Part model, mm, in its own coordinate system. Coordinates: 2 decimals unless noted, no trailing zeros. Write each loop counter-clockwise with the first axis right and the second up, starting at its lowest first coordinate (ties: lowest second). Pieces come first, ordered by that corner, then holes. Notation, with made-up numbers: M 52.25,64 L 56.25,64 A21 cw 56.25,85 Z; hole C 0,66 d3. An arc over 180 degrees is marked long. Use a Markdown table: item, result. Add a question column.
Q1. Slice it at A-A on y = -25. Write the cut outline in (x, z) (3 decimals), then the cut area to 3 significant figures.
Q2. Pin check, flat tips, straight feed: pin 1 Ø1.6 at (x, z) = (0.5, 2) entering from +Y; pin 2 Ø1.6 at (y, z) = (-39, 1) entering from +X; pin 3 Ø1 at (y, z) = (65, 1.5) entering from -X; pin 4 Ø10 at (x, y) = (7, 2.5) entering from -Z. Stop position of each tip, or through.
Q3. Wall check: L1, parallel to Y at x = 30, z = 0.8; L2, parallel to Y at x = -22, z = 1.8; L3, parallel to Y at x = 17, z = 2. Give the ranges that are in metal, low to high. Write a range as from..to.
Q4. Slice it at C-C on y = 33.5. Write the cut outline in (x, z) (3 decimals).
Q5. Slice it at B-B on x = 33. Write the cut outline in (y, z) (3 decimals), then the cut area to 3 significant figures.
Q6. Slice it at D-D on z = 2.3. Count the separate pieces of the cut face and the enclosed holes in it, then the cut area to 3 significant figures.
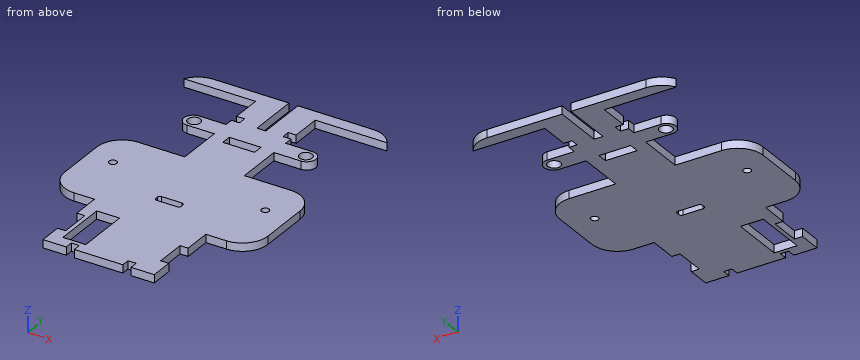
from build123d import *

# Parameters (mm, degrees)
SKETCH1_R           = 2.5
BOSS_EXTRUDE1_DEPTH = 3.175
FILLET1_R           = 10
SKETCH2_W           = 9
SKETCH2_H           = 21
CUT_EXTRUDE1_DEPTH  = 90.108082017
SKETCH3_W           = 12.5
SKETCH3_H           = 4
SKETCH3_W_2         = 3.5
SKETCH3_H_2         = 20
CUT_EXTRUDE2_DEPTH  = 90.108082017
FILLET2_R           = 10
SKETCH4_W           = 3.175
SKETCH4_H           = 3.175
BOSS_EXTRUDE2_DEPTH = 29
SKETCH5_W           = 3.175
SKETCH5_H           = 3.175
BOSS_EXTRUDE3_DEPTH = 29
SKETCH7_R           = 1.5
CUT_EXTRUDE3_DEPTH  = 10


with BuildPart() as part:
    # Sketch1 → Boss-Extrude1 (new body)
    with BuildSketch(Plane.XY):
        with BuildLine():
            Line((-9.56, -38.262636689), (-9.56, -41.437636689))
            Line((-9.56, -41.437636689), (9.56, -41.437636689))
            Line((9.56, -41.437636689), (9.56, -38.262636689))
            Line((9.56, -38.262636689), (12.735, -38.262636689))
            Line((12.735, -38.262636689), (12.735, -41.437636689))
            Line((12.735, -41.437636689), (15.91, -41.437636689))
            Line((15.91, -41.437636689), (21.91, -41.437636689))
            Line((21.91, -41.437636689), (21.91, -32.437636689))
            Line((21.91, -32.437636689), (18.735, -32.437636689))
            Line((18.735, -32.437636689), (18.735, -20.437636689))
            Line((18.735, -20.437636689), (21.91, -20.437636689))
            Line((21.91, -20.437636689), (21.91, -9.437636689))
            Line((21.91, -9.437636689), (40, -9.437636689))
            Line((40, -9.437636689), (40, 30.562363311))
            Line((40, 30.562363311), (10, 30.562363311))
            Line((10, 30.562363311), (10, 45.562363311))
            Line((10, 45.562363311), (10, 48.89577614))
            Line((10, 48.89577614), (22.410269523, 48.89577614))
            ThreePointArc((22.410269523, 48.89577614), (26.000000001, 52.562363311), (22.410269523, 56.228950483))
            Line((22.410269523, 56.228950483), (11.727794547, 56.228950483))
            Line((11.727794547, 56.228950483), (11.727794547, 59.562363311))
            Line((11.727794547, 59.562363311), (10, 59.562363311))
            Line((10, 59.562363311), (8.552794547, 59.562363311))
            Line((8.552794547, 59.562363311), (8.552794547, 62.737363311))
            Line((8.552794547, 62.737363311), (11.727794547, 62.737363311))
            Line((11.727794547, 62.737363311), (11.727794547, 74.562363311))
            Line((11.727794547, 74.562363311), (40, 74.562363311))
            Line((40, 74.562363311), (40, 79.562363311))
            Line((40, 79.562363311), (0, 79.562363311))
            Line((0, 79.562363311), (-40, 79.562363311))
            Line((-40, 79.562363311), (-40, 74.562363311))
            Line((-40, 74.562363311), (-11.727794547, 74.562363311))
            Line((-11.727794547, 74.562363311), (-11.727794547, 62.737363311))
            Line((-11.727794547, 62.737363311), (-8.552794547, 62.737363311))
            Line((-8.552794547, 62.737363311), (-8.552794547, 59.562363311))
            Line((-8.552794547, 59.562363311), (-10, 59.562363311))
            Line((-10, 59.562363311), (-11.727794547, 59.562363311))
            Line((-11.727794547, 59.562363311), (-11.727794547, 56.228950483))
            Line((-11.727794547, 56.228950483), (-22.410269523, 56.228950483))
            ThreePointArc((-22.410269523, 56.228950483), (-26.000000001, 52.562363311), (-22.410269523, 48.89577614))
            Line((-22.410269523, 48.89577614), (-10, 48.89577614))
            Line((-10, 48.89577614), (-10, 45.562363311))
            Line((-10, 45.562363311), (-10, 30.562363311))
            Line((-10, 30.562363311), (-40, 30.562363311))
            Line((-40, 30.562363311), (-40, -9.437636689))
            Line((-40, -9.437636689), (-21.91, -9.437636689))
            Line((-21.91, -9.437636689), (-21.91, -20.437636689))
            Line((-21.91, -20.437636689), (-18.735, -20.437636689))
            Line((-18.735, -20.437636689), (-18.735, -32.437636689))
            Line((-18.735, -32.437636689), (-21.91, -32.437636689))
            Line((-21.91, -32.437636689), (-21.91, -41.437636689))
            Line((-21.91, -41.437636689), (-15.91, -41.437636689))
            Line((-15.91, -41.437636689), (-12.735, -41.437636689))
            Line((-12.735, -41.437636689), (-12.735, -38.262636689))
            Line((-12.735, -38.262636689), (-9.56, -38.262636689))
        make_face()
        with BuildLine():
            Line((4, 1), (-4, 1))
            ThreePointArc((-4, 1), (-4.707106781, 1.292893219), (-5, 2))
            Line((-5, 2), (-5, 3))
            ThreePointArc((-5, 3), (-4.707106781, 3.707106781), (-4, 4))
            Line((-4, 4), (4, 4))
            ThreePointArc((4, 4), (4.707106781, 3.707106781), (5, 3))
            Line((5, 3), (5, 2))
            ThreePointArc((5, 2), (4.707106781, 1.292893219), (4, 1))
        make_face(mode=Mode.SUBTRACT)
        with Locations((-22, 52.562363311)):
            Circle(SKETCH1_R, mode=Mode.SUBTRACT)
        with Locations((22, 52.562363311)):
            Circle(SKETCH1_R, mode=Mode.SUBTRACT)
    extrude(amount=BOSS_EXTRUDE1_DEPTH)

    # Fillet1
    # the kernel refuses this fillet: 10 mm, written as the material it takes off along each edge
    with BuildSketch(Plane(origin=(-40, 79.562363311, -21.650635095), x_dir=(0, -1, 0), z_dir=(0, 0, 1))) as fillet1_piece_1:
        with BuildLine():
            CenterArc((10, 8.660254038), FILLET1_R, 180, 60)
            Line((0, 8.660254038), (-0.2, 8.660254038))
            Line((-0.2, 8.660254038), (-0.2, 0))
            Line((-0.2, 0), (0, -0.2))
            ThreePointArc((0, -0.2), (2.5, -0.2), (4.9, -0.173205081))
            Line((4.9, -0.173205081), (5, 0))
        make_face()
    extrude(amount=46.476270189, mode=Mode.SUBTRACT)
    with BuildSketch(Plane(origin=(40, 79.562363311, -21.650635095), x_dir=(-1, 0, 0), z_dir=(0, 0, 1))) as fillet1_piece_2:
        with BuildLine():
            CenterArc((8.660254038, 10), FILLET1_R, 210, 60)
            Line((0, 5), (-0.173205081, 4.9))
            ThreePointArc((-0.173205081, 4.9), (-0.2, 2.5), (-0.2, 0))
            Line((-0.2, 0), (0, -0.2))
            Line((0, -0.2), (8.660254038, -0.2))
            Line((8.660254038, -0.2), (8.660254038, 0))
        make_face()
    extrude(amount=46.476270189, mode=Mode.SUBTRACT)

    # Sketch2 → Cut-Extrude1 (cut, through all)
    with BuildSketch(Plane.XY.offset(3.175)):
        with Locations((-12.61, -26.137636689)):
            Rectangle(SKETCH2_W, SKETCH2_H)
    extrude(amount=-CUT_EXTRUDE1_DEPTH, mode=Mode.SUBTRACT)

    # Sketch3 → Cut-Extrude2 (cut, through all)
    with BuildSketch(Plane.XY.offset(3.175)):
        with Locations((0, 47.562363311)):
            Rectangle(SKETCH3_W, SKETCH3_H)
        with Locations((0, 69.663077344)):
            Rectangle(SKETCH3_W_2, SKETCH3_H_2)
    extrude(amount=-CUT_EXTRUDE2_DEPTH, mode=Mode.SUBTRACT)

    # Fillet2
    fillet2_edges = [part.edges().sort_by_distance(p)[0] for p in [
        (40, 30.562363311, 1.5875),
        (40, -9.437636689, 1.5875),
        (-40, -9.437636689, 1.5875),
        (-40, 30.562363311, 1.5875),
    ]]
    fillet(fillet2_edges, radius=FILLET2_R)

    # Sketch4 → Boss-Extrude2 (add)
    with BuildSketch(Plane(origin=(0, 59.562363311, 0), x_dir=(1, 0, 0), z_dir=(0, 1, 0))):
        with Locations((10.140294547, -1.5875)):
            Rectangle(SKETCH4_W, SKETCH4_H)
    extrude(amount=-BOSS_EXTRUDE2_DEPTH)

    # Sketch5 → Boss-Extrude3 (add)
    with BuildSketch(Plane(origin=(0, 59.562363311, 0), x_dir=(1, 0, 0), z_dir=(0, 1, 0))):
        with Locations((-10.140294547, -1.5875)):
            Rectangle(SKETCH5_W, SKETCH5_H)
    extrude(amount=-BOSS_EXTRUDE3_DEPTH)

    # Sketch7 → Cut-Extrude3 (cut)
    with BuildSketch(Plane.XY.offset(3.175)):
        with Locations((-30, 14.733489054)):
            Circle(SKETCH7_R)
        with Locations((30, 14.733489054)):
            Circle(SKETCH7_R)
    extrude(amount=-CUT_EXTRUDE3_DEPTH, mode=Mode.SUBTRACT)


solid = part.part
Recorded:
| question | item | result |
|---|---|---|
| 1 | outline | M -18.735,0 L -17.11,0 L -17.11,3.175 L -18.735,3.175 Z; M -8.11,0 L 18.735,0 L 18.735,3.175 L -8.11,3.175 Z |
| 1 | area | 90.4 mm² |
| 2 | pin 1 | y = 59.66 |
| 2 | pin 2 | x = 21.91 |
| 2 | pin 3 | x = -11.73 |
| 2 | pin 4 | z = 0 |
| 3 | L1 | -9.44..13.23, 16.23..30.56, 74.56..79.56 |
| 3 | L2 | -9.44..30.56, 48.9..50.06, 55.06..56.23, 74.56..79.56 |
| 3 | L3 | -41.44..30.56, 48.9..56.23, 74.56..79.56 |
| 4 | outline | M -11.728,0 L 11.728,0 L 11.728,3.175 L -11.728,3.175 Z |
| 5 | outline | M -8.977,0 L 30.102,0 L 30.102,3.175 L -8.977,3.175 Z; M 74.562,0 L 79.424,0 L 79.424,3.175 L 74.562,3.175 Z |
| 5 | area | 140 mm² |
| 6 | separate pieces | 1 |
| 6 | enclosed holes | 7 |
| 6 | area | 5,610 mm² |
